Autodesk Inventor part; units mm, degrees
ref_plane "YZ Plane" through (0, 0, 0) normal (1, 0, 0) x (0, 1, 0)
ref_plane "XZ Plane" through (0, 0, 0) normal (0, 1, 0) x (-1, 0, 0)
ref_plane "XY Plane" through (0, 0, 0) normal (0, 0, 1) x (1, 0, 0)
sketch "Sketch1" plane through (0, 0, 0) normal (0, 1, 0) x (-1, 0, 0)
  line L0 (0, 0) -> (0, -42)
  line L1 (0, -42) -> (42, -42)
  line L2 (42, -42) -> (42, 0)
  line L3 (42, 0) -> (0, 0)
  line L4 (0, 0) -> (42, 0)
  dimension "d0" = 42
  dimension "d1" = 42
extrude "Extrusion1" add sketch "Sketch1" along normal blind 39
sketch "Sketch2" plane through (0, 39, 0) normal (0, 1, 0) x (1, 0, 0)
  line L0 (0, 0) -> (0, 42)
  line L1 (-41.7664, 0) -> (0, 42)
  circle A0 centre (-20.8832, 21) radius 11
  dimension "d4" = 22
extrude "Extrusion2" add sketch "Sketch2" along normal blind 2
sketch "Sketch3" plane through (-20.8832, 41, -21) normal (0, 1, 0) x (1, 0, 0)
  circle A0 centre (0, 0) radius 2.5
  point P0 (20.8832, -21)
  dimension "d7" = 5
extrude "Extrusion3" add sketch "Sketch3" along normal blind 22
properties part number "motor"
Build history of the part. All positions in model axes, mm. A direction names the side the tool comes from. Round coordinates to 2 decimals unless told otherwise and drop trailing zeros. Order: outer loops, then holes, each group sorted by start corner. A loop starts at its lowest first (then second) coordinate and runs counter-clockwise, first axis right, second up. Notation, with made-up numbers: (-20, 28) -> (-7, 28) arc R28 ccw to (-7, 67) -> close; hole circle Ø9 at (-26.75, 34). An arc over 180 degrees is marked (long way). Answer in a Markdown table with one row per item.
1) Which spindle directions (+Z, -Z, +X, -X, +Y, -Y) get a long thin tool onto all of the face, cutting with end or side? Do faces 1 (the flat face through (-30, 39, -30)), 2 (the flat face through (-21, 19, 0)). Say none if no direction does.
Values:
| item | result |
|---|---|
| face 1 | +Y |
| face 2 | +Z, +X, -X, +Y, -Y |
2) Band-saw the part on B-B on x = -21. Give the cut face in (y, z).
Values:
| item | result |
|---|---|
| outline | (0, -42) -> (39, -42) -> (39, -32) -> (41, -32) -> (41, -23.5) -> (63, -23.5) -> (63, -18.5) -> (41, -18.5) -> (41, -10) -> (39, -10) -> (39, 0) -> (0, 0) -> close |
3) Band-saw the part on D-D on z = -29. Give the cut face in (x, y).
Values:
| item | result |
|---|---|
| outline | (-42, 0) -> (0, 0) -> (0, 39) -> (-13.33, 39) -> (-13.33, 41) -> (-28.43, 41) -> (-28.43, 39) -> (-42, 39) -> close |
4) Pin check, flat tip, straight feed: P1, Ø6, axis at x = -14, z = -21, coming from the +Y side. Stop position of the tip, or through.
Values:
| item | result |
|---|---|
| P1 | y = 41 |
5) Band-saw the part on C-C on y = 46. Give the cut face in (x, z), and give its area (3 significant figures).
Values:
| item | result |
|---|---|
| outline | circle Ø5 at (-20.88, -21) |
| area | 19.6 mm2 |
6) Wall check: L1, parallel to Y at x = -4.5, z = -25; L2, parallel to Y at x = -11.5, z = -23; L3, parallel to Z at x = -23, y = 52. Give the ranges that are in metal, low to high.
Values:
| item | result |
|---|---|
| L1 | 0 to 39 |
| L2 | 0 to 41 |
| L3 | -22.33 to -19.67 |
7) Band-saw the part on A-A on z = -21. Give the cut face in (x, y).
Values:
| item | result |
|---|---|
| outline | (-42, 0) -> (0, 0) -> (0, 39) -> (-9.88, 39) -> (-9.88, 41) -> (-18.38, 41) -> (-18.38, 63) -> (-23.38, 63) -> (-23.38, 41) -> (-31.88, 41) -> (-31.88, 39) -> (-42, 39) -> close |
